Source: three-view drawing plus pictorial views. Frame: mm from the lowest corner of the part. Round coordinates to 2 decimals unless told otherwise and drop trailing zeros. Write each loop counter-clockwise with the first axis right and the second up, starting at its lowest first coordinate (ties: lowest second). Pieces come first, ordered by that corner, then holes. Notation, with made-up numbers: M -4.75,-39 L -0.75,-39 A27 cw -0.75,-12 Z; hole C 81.5,66.25 d5. An arc over 180 degrees is marked long. Answer in a Markdown table with one row per item.
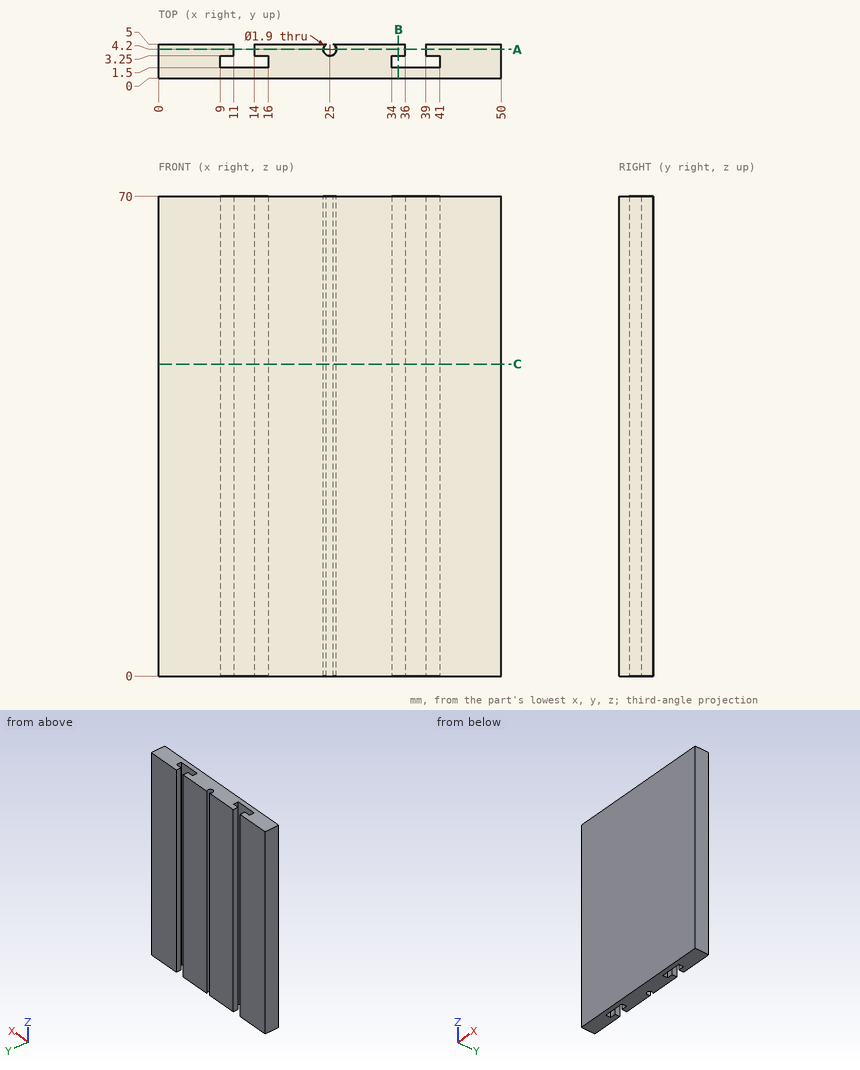
Q1. Material intervals for probe 1 along X at (y, z) = (4.2, 46); probe 2 along X at (y, z) = (2.7, 36.5); probe 3 along Y at (x, z) = (40, 58.5), sorted ascending.
Solutions:
| item | result |
|---|---|
| probe 1 | x = 0 to 11, 14 to 24.05, 25.95 to 36, 39 to 50 |
| probe 2 | x = 0 to 9, 16 to 34, 41 to 50 |
| probe 3 | y = 0 to 1.5, 3.25 to 5 |
Q2. Section A-A (y = 4.2). Return loops of the section in (x, z), and give its area (3 significant figures).
Solutions:
| item | result |
|---|---|
| outline | M 0,0 L 11,0 L 11,70 L 0,70 Z; M 14,0 L 24.05,0 L 24.05,70 L 14,70 Z; M 25.95,0 L 36,0 L 36,70 L 25.95,70 Z; M 39,0 L 50,0 L 50,70 L 39,70 Z |
| area | 2,950 mm2 |
Q3. Section C-C (z = 45.5). Return loops of the section in (x, y), and give its area (3 significant figures).
Solutions:
| item | result |
|---|---|
| outline | M 0,0 L 50,0 L 50,5 L 39,5 L 39,3.25 L 41,3.25 L 41,1.5 L 34,1.5 L 34,3.25 L 36,3.25 L 36,5 L 25.51,5 A0.95 cw long 24.49,5 L 14,5 L 14,3.25 L 16,3.25 L 16,1.5 L 9,1.5 L 9,3.25 L 11,3.25 L 11,5 L 0,5 Z |
| area | 212 mm2 |
Q4. Section B-B (x = 35). Return loops of the section in (y, z), and give its area (4 significant figures).
Solutions:
| item | result |
|---|---|
| outline | M 0,0 L 1.5,0 L 1.5,70 L 0,70 Z; M 3.25,0 L 5,0 L 5,70 L 3.25,70 Z |
| area | 227.5 mm2 |
